from build123d import *

# Parameters (mm, degrees)
SKETCH1_W           = 95
SKETCH1_H           = 95
BOSS_EXTRUDE1_DEPTH = 20
FILLET1_R           = 10
CUT_EXTRUDE5_DEPTH  = 18.5
CUT_EXTRUDE6_DEPTH  = 10
SKETCH6_W           = 13.621181439
SKETCH6_H           = 6.835350155
CUT_EXTRUDE7_DEPTH  = 10
SKETCH9_W           = 10.583669907
SKETCH9_H           = 4.379449617
CUT_EXTRUDE10_DEPTH = 10


with BuildPart() as part:
    # Sketch1 → Boss-Extrude1 (new body)
    with BuildSketch(Plane(origin=(0, 0, 0), x_dir=(1, 0, 0), z_dir=(0, 1, 0))):
        Rectangle(SKETCH1_W, SKETCH1_H)
    extrude(amount=BOSS_EXTRUDE1_DEPTH)

    # Fillet1
    fillet1_edges = [part.edges().sort_by_distance(p)[0] for p in [
        (47.5, 10, 47.5),
        (-47.5, 10, 47.5),
        (-47.5, 10, -47.5),
        (47.5, 10, -47.5),
    ]]
    fillet(fillet1_edges, radius=FILLET1_R)

    # Sketch4 → Cut-Extrude5 (cut)
    with BuildSketch(Plane(origin=(0, 20, 0), x_dir=(1, 0, 0), z_dir=(0, 1, 0))):
        with BuildLine():
            Line((37.5, 46), (-37.5, 46))
            ThreePointArc((-37.5, 46), (-43.51040764, 43.51040764), (-46, 37.5))
            Line((-46, 37.5), (-46, -37.5))
            ThreePointArc((-46, -37.5), (-43.51040764, -43.51040764), (-37.5, -46))
            Line((-37.5, -46), (37.5, -46))
            ThreePointArc((37.5, -46), (43.51040764, -43.51040764), (46, -37.5))
            Line((46, -37.5), (46, 37.5))
            ThreePointArc((46, 37.5), (43.51040764, 43.51040764), (37.5, 46))
        make_face()
    extrude(amount=-CUT_EXTRUDE5_DEPTH, mode=Mode.SUBTRACT)

    # Sketch5 → Cut-Extrude6 (cut)
    with BuildSketch(Plane.ZY.offset(47.5)):
        with BuildLine():
            Line((-32.917062514, 13.76355051), (-26.545864744, 13.76355051))
            ThreePointArc((-26.545864744, 13.76355051), (-24.370980604, 11.588666369), (-26.545864744, 9.413782229))
            Line((-26.545864744, 9.413782229), (-32.917062514, 9.413782229))
            ThreePointArc((-32.917062514, 9.413782229), (-35.091946654, 11.588666369), (-32.917062514, 13.76355051))
        make_face()
    extrude(amount=-CUT_EXTRUDE6_DEPTH, mode=Mode.SUBTRACT)

    # Sketch6 → Cut-Extrude7 (cut)
    with BuildSketch(Plane.ZY.offset(47.5)):
        with Locations((-9.409539708, 11.899364103)):
            Rectangle(SKETCH6_W, SKETCH6_H)
    extrude(amount=-CUT_EXTRUDE7_DEPTH, mode=Mode.SUBTRACT)

    # Sketch9 → Cut-Extrude10 (cut)
    with BuildSketch(Plane.XY.offset(47.5)):
        with Locations((-1.457227674, 4.56970852)):
            Rectangle(SKETCH9_W, SKETCH9_H)
        with Locations((-1.457227674, 12.233745351)):
            Rectangle(SKETCH9_W, SKETCH9_H)
    extrude(amount=-CUT_EXTRUDE10_DEPTH, mode=Mode.SUBTRACT)


solid = part.part
Input: part model. Units: mm. Frame: model coordinates. A direction names the side the tool comes from. Coordinates: 2 decimals unless noted, no trailing zeros. Loops run counter-clockwise (first coordinate to the right, second up) from the corner with the lowest first, then second, coordinate; pieces in that order, holes last.
Q1. Contact query for flat-ended pins moving along their axis: pin 1 (0.8 mm diameter, centred on y = 4, z = 46.5, fed in from -X); pin 2 (12 mm diameter, centred on x = -23.5, z = -20.5, fed in from -Y); pin 3 (10 mm diameter, centred on x = 21.5, z = 23.5, fed in from +Y); pin 4 (1.2 mm diameter, centred on y = 12.5, z = 47, fed in from +X). Output: stop coordinate, or through.
Q2. Cut plane B-B (z = -28). Output: boundary loops of the cut face in (x, y).
Q3. Draft query along Z for faces 1 (the face through (47.5, 10, 1)), 2 (the face through (-1, 10, -47.5)), 3 (the face through (-1, 9, 46)), 4 (the face through (43.58, 10.88, -43.44)). Return one class per face: +Z half, -Z half, draft (parallel to the pull), parting line (faces both ways), or undercut.
Q4. Cut plane A-A (y = 17). Output: boundary loops of the cut face in (x, z).
Q5. Material intervals for line 1 (Z direction, x = 1.5, y = 15); line 2 (Y direction, x = 31.5, z = -2), sorted ascending.
Q6. Cut plane C-C (y = 11.75). Output: boundary loops of the cut face in (x, z), then the cut area to 3 significant figures.
Q7. Cut plane D-D (z = 0). Output: boundary loops of the cut face in (x, y).
Q8. Set-up query: faces 5 (the face through (-46.76, 11.54, -35.09)), 6 (the face through (1, 11, -46)), 7 (the face through (-46, 20, -42)). Return all of +Z, -Z, +X, -X, +Y, -Y with unobstructed straight access to the full face (end or side cutting, diameter ignored); none if empty.
Working result:
1. pin 1: stops at x = -42.6
1. pin 2: stops at y = 0
1. pin 3: stops at y = 1.5
1. pin 4: stops at x = 42.06
2. outline: (-47.5, 0) - (47.5, 0) - (47.5, 20) - (46, 20) - (46, 1.5) - (-46, 1.5) - (-46, 9.41) - (-47.5, 9.41) - close; (-47.5, 13.76) - (-46, 13.76) - (-46, 20) - (-47.5, 20) - close
3. face 1: draft
3. face 2: -Z half
3. face 3: undercut
3. face 4: undercut
4. outline: (-47.5, -37.5) arc R10 ccw to (-37.5, -47.5) - (37.5, -47.5) arc R10 ccw to (47.5, -37.5) - (47.5, 37.5) arc R10 ccw to (37.5, 47.5) - (-37.5, 47.5) arc R10 ccw to (-47.5, 37.5) - close; hole (-46, -37.5) arc R8.5 ccw to (-37.5, -46) - (37.5, -46) arc R8.5 ccw to (46, -37.5) - (46, 37.5) arc R8.5 ccw to (37.5, 46) - (-37.5, 46) arc R8.5 ccw to (-46, 37.5) - close
5. line 1: z = -47.5 to -46, 46 to 47.5
5. line 2: y = 0 to 1.5
6. outline: (-47.5, -37.5) arc R10 ccw to (-37.5, -47.5) - (37.5, -47.5) arc R10 ccw to (47.5, -37.5) - (47.5, 37.5) arc R10 ccw to (37.5, 47.5) - (3.83, 47.5) - (3.83, 46) - (37.5, 46) arc R8.5 cw to (46, 37.5) - (46, -37.5) arc R8.5 cw to (37.5, -46) - (-37.5, -46) arc R8.5 cw to (-46, -37.5) - (-46, -35.09) - (-47.5, -35.09) - close; (-47.5, -24.38) - (-46, -24.38) - (-46, -16.22) - (-47.5, -16.22) - close; (-47.5, -2.6) - (-46, -2.6) - (-46, 37.5) arc R8.5 cw to (-37.5, 46) - (-6.75, 46) - (-6.75, 47.5) - (-37.5, 47.5) arc R10 ccw to (-47.5, 37.5) - close
6. area: 485 mm2
7. outline: (-47.5, 0) - (47.5, 0) - (47.5, 20) - (46, 20) - (46, 1.5) - (-46, 1.5) - (-46, 20) - (-47.5, 20) - close
8. face 5: -X
8. face 6: +Y
8. face 7: +Z, -Z, +X, -X, +Y
